Input: part model. Units: mm. Frame: model coordinates. A direction names the side the tool comes from. Round coordinates to 2 decimals unless told otherwise and drop trailing zeros. Write each loop counter-clockwise with the first axis right and the second up, starting at its lowest first coordinate (ties: lowest second). Pieces come first, ordered by that corner, then holes. Notation, with made-up numbers: (85, 58) -> (126, 58) arc R23 ccw to (126, 80) -> close; hole circle Ø11 at (79.5, 31.5). An arc over 180 degrees is marked (long way). Use CSV: the item, a comma, the result in double quotes.
```python
from build123d import *

# Parameters (mm, degrees)
ESQUISSE1_W             = 125
ESQUISSE1_H             = 80
BOSS_EXTRU_1_DEPTH      = 3
ESQUISSE2_W             = 125
ESQUISSE2_H             = 103.25
BOSS_EXTRU_2_DEPTH      = 3
ESQUISSE6_W             = 5
ESQUISSE6_H             = 3.5
BOSS_EXTRU_5_DEPTH      = 125
ESQUISSE7_R             = 2.5
ENL_V_MAT_EXTRU_2_DEPTH = 3


with BuildPart() as part:
    # Esquisse1 → Boss.-Extru.1 (new body)
    with BuildSketch(Plane(origin=(0, 0, 0), x_dir=(1, 0, 0), z_dir=(0, 1, 0))):
        with Locations((52.5, 25.1)):
            Rectangle(ESQUISSE1_W, ESQUISSE1_H)
        with BuildLine():
            ThreePointArc((10.2, 0), (5.1, -5.1), (0, 0))
            Line((0, 0), (0, 50.2))
            ThreePointArc((0, 50.2), (5.1, 55.3), (10.2, 50.2))
            Line((10.2, 50.2), (10.2, 0))
        make_face(mode=Mode.SUBTRACT)
    boss_extru_1 = extrude(amount=BOSS_EXTRU_1_DEPTH)

    # Esquisse2 → Boss.-Extru.2 (add)
    with BuildSketch(Plane(origin=(0, 0, -65.1), x_dir=(-1, 0, 0), z_dir=(0, 0, -1))):
        with Locations((-52.5, -48.625)):
            Rectangle(ESQUISSE2_W, ESQUISSE2_H)
    extrude(amount=BOSS_EXTRU_2_DEPTH)

    # Symétrie1: Boss.-Extru.1 across plane
    add(boss_extru_1.mirror(Plane(origin=(0, -48.625, 0), x_dir=(0, 0, 1), z_dir=(0, -1, 0))))

    # Esquisse6 → Boss.-Extru.5 (add)
    with BuildSketch(Plane(origin=(115, 0, 0), x_dir=(0, 0, -1), z_dir=(1, 0, 0))):
        with Locations((-12.4, -95.5)):
            Rectangle(ESQUISSE6_W, ESQUISSE6_H)
        with Locations((-12.4, -102)):
            Rectangle(ESQUISSE6_W, ESQUISSE6_H)
        Polygon((-14.9, -103.75), (-9.9, -103.75), (-14.9, -108.75), align=None)
        Polygon((-14.9, -93.75), (-14.9, -88.75), (-9.9, -93.75), align=None)
        Polygon((-14.9, -3.5), (-14.9, -8.5), (-9.9, -3.5), align=None)
        with Locations((-12.4, -1.75)):
            Rectangle(ESQUISSE6_W, ESQUISSE6_H)
        with Locations((-12.4, 4.75)):
            Rectangle(ESQUISSE6_W, ESQUISSE6_H)
        Polygon((-14.9, 11.5), (-9.9, 6.5), (-14.9, 6.5), align=None)
    extrude(amount=-BOSS_EXTRU_5_DEPTH)

    # Esquisse7 → Enlèv. mat.-Extru.2 (cut)
    with BuildSketch(Plane(origin=(0, 0, -68.1), x_dir=(-1, 0, 0), z_dir=(0, 0, -1))):
        with Locations((-90, -17)):
            Circle(ESQUISSE7_R)
        with Locations((-75, -17)):
            Circle(ESQUISSE7_R)
        with Locations((-60, -17)):
            Circle(ESQUISSE7_R)
        with Locations((-45, -17)):
            Circle(ESQUISSE7_R)
        with Locations((-30, -17)):
            Circle(ESQUISSE7_R)
        with Locations((-15, -17)):
            Circle(ESQUISSE7_R)
        with Locations((-75, -47)):
            Circle(ESQUISSE7_R)
        with Locations((-60, -47)):
            Circle(ESQUISSE7_R)
        with Locations((-45, -47)):
            Circle(ESQUISSE7_R)
        with Locations((-30, -47)):
            Circle(ESQUISSE7_R)
        with Locations((-15, -47)):
            Circle(ESQUISSE7_R)
        with Locations((-75, -77)):
            Circle(ESQUISSE7_R)
        with Locations((-60, -77)):
            Circle(ESQUISSE7_R)
        with Locations((-45, -77)):
            Circle(ESQUISSE7_R)
        with Locations((-30, -77)):
            Circle(ESQUISSE7_R)
        with Locations((-15, -77)):
            Circle(ESQUISSE7_R)
        with Locations((-90, -47)):
            Circle(ESQUISSE7_R)
        with Locations((-90, -77)):
            Circle(ESQUISSE7_R)
    extrude(amount=-ENL_V_MAT_EXTRU_2_DEPTH, mode=Mode.SUBTRACT)


solid = part.part
```
Item 1: First-contact query: pin 1 Ø6 at (x, z) = (58.5, -30) entering from +Y; pin 2 Ø6 at (x, y) = (75, -47) entering from +Z; pin 3 Ø1 at (x, y) = (24.5, -102.5) entering from -Z. Flat tips, straight axial feed; report the tip coordinate or a pass-through.
Worked answers:
pin 1,"stops at y = 3"
pin 2,"stops at z = -65.1"
pin 3,"stops at z = 9.9"
Item 2: Set-up query: faces 1 (the face through (53, -48, -65.1)), 2 (the face through (53, 3, -29)), 3 (the face through (53, -102, 9.9)). Return all of +Z, -Z, +X, -X, +Y, -Y with unobstructed straight access to the full face (end or side cutting, diameter ignored); none if empty.
Worked answers:
face 1,"+X, -X"
face 2,"-Z, +X, -X, +Y"
face 3,"-Z, +X, -X, -Y"
Item 3: Section query A-A on z = -60. Return the cut outline in (x, y).
Worked answers:
outline,"(-10, -100.25) -> (115, -100.25) -> (115, -97.25) -> (-10, -97.25) -> close; (-10, 0) -> (115, 0) -> (115, 3) -> (-10, 3) -> close"
Item 4: Section query D-D on z = -44.5. Return the cut outline in (x, y), plus the area to 3 significant figures.
Worked answers:
outline,"(-10, -100.25) -> (0, -100.25) -> (0, -97.25) -> (-10, -97.25) -> close; (-10, 0) -> (0, 0) -> (0, 3) -> (-10, 3) -> close; (10.2, -100.25) -> (115, -100.25) -> (115, -97.25) -> (10.2, -97.25) -> close; (10.2, 0) -> (115, 0) -> (115, 3) -> (10.2, 3) -> close"
area,"689 mm²"
Item 5: Section query B-B on x = 30. Return the cut outline in (y, z).
Worked answers:
outline,"(-108.75, 14.9) -> (-103.75, 9.9) -> (-100.25, 9.9) -> (-100.25, -68.1) -> (-79.5, -68.1) -> (-79.5, -65.1) -> (-97.25, -65.1) -> (-97.25, 9.9) -> (-93.75, 9.9) -> (-88.75, 14.9) -> close; (-74.5, -68.1) -> (-49.5, -68.1) -> (-49.5, -65.1) -> (-74.5, -65.1) -> close; (-44.5, -68.1) -> (-19.5, -68.1) -> (-19.5, -65.1) -> (-44.5, -65.1) -> close; (-14.5, -68.1) -> (3, -68.1) -> (3, 9.9) -> (6.5, 9.9) -> (11.5, 14.9) -> (-8.5, 14.9) -> (-3.5, 9.9) -> (0, 9.9) -> (0, -65.1) -> (-14.5, -65.1) -> close"
Item 6: Line query: line 1 (Y direction, x = 75, z = -66.9); line 2 (Y direction, x = 68, z = -10); line 3 (Z direction, x = 103.5, y = -96). Output: solid intervals per line, ascending.
Worked answers:
line 1,"y = -100.25 to -79.5, -74.5 to -49.5, -44.5 to -19.5, -14.5 to 3"
line 2,"y = -100.25 to -97.25, 0 to 3"
line 3,"z = -68.1 to -65.1, 9.9 to 14.9"
Item 7: Pull-direction query (Z, two-part tool) for faces 4 (the face through (53, -48, -68.1)), 5 (the face through (92, -48.5, -66.6)), 6 (the face through (53, -96, 9.9)); classes: +Z half, -Z half, draft (parallel to the pull), parting line (faces both ways), or undercut.
Worked answers:
face 4,"-Z half"
face 5,"draft"
face 6,"undercut"
Item 8: Section query C-C on y = -47. Return the cut outline in (x, z).
Worked answers:
outline,"(-10, -68.1) -> (12.5, -68.1) -> (12.5, -65.1) -> (-10, -65.1) -> close; (17.5, -68.1) -> (27.5, -68.1) -> (27.5, -65.1) -> (17.5, -65.1) -> close; (32.5, -68.1) -> (42.5, -68.1) -> (42.5, -65.1) -> (32.5, -65.1) -> close; (47.5, -68.1) -> (57.5, -68.1) -> (57.5, -65.1) -> (47.5, -65.1) -> close; (62.5, -68.1) -> (72.5, -68.1) -> (72.5, -65.1) -> (62.5, -65.1) -> close; (77.5, -68.1) -> (87.5, -68.1) -> (87.5, -65.1) -> (77.5, -65.1) -> close; (92.5, -68.1) -> (115, -68.1) -> (115, -65.1) -> (92.5, -65.1) -> close"
